The model under review builds one solid part; all positions refer to its coordinate system, in mm. A direction names the side the tool comes from. Round coordinates to 2 decimals unless told otherwise and drop trailing zeros. Order: outer loops, then holes, each group sorted by start corner. A loop starts at its lowest first (then second) coordinate and runs counter-clockwise, first axis right, second up. Notation, with made-up numbers: M 22.25,0 L 36.25,0 A17 cw 36.25,18 Z; hole C 81,37.5 d9. An arc over 180 degrees is marked long. Answer as a JSON object with one key per item and string values. Group by question number.
1) The part is to be moulded in two halves that separate along X. For faces 1 (the flat face through (-26.358, -0.239, 43.368)), 2 (the flat face through (27.625, 0, 25)), 3 (the cylindrical face through (28.62, -23.45, 27.78)), 4 (the flat face through (28, 0, 0)), say which applies: +X half, -X half, draft (parallel to the pull), parting line (faces both ways), or undercut.
2) To check wall thickness, follow line 1 (X direction, y = 12, z = 36) (3 decimals); line 2 (X direction, y = -14, z = 46) (3 decimals); line 3 (Y direction, x = 25.5, z = 9). State the ranges of each line that lie inside material, in increasing order.
3) For faces 5 (the flat face through (14, 21, 52.3)), 6 (the flat face through (25.125, -22, 25)), 7 (the flat face through (26, 17.05, 25)), 8 (the flat face through (0, 0, 54.8)), list the 3-axis set-ups (+Z, -Z, +X, -X, +Y, -Y) from which the entire face can be reached by the end or side of a thin tool; tool diameter is ignored.
4) Consider section C-C, the plane x = -3. Write out the cut boundary in (y, z) (3 decimals).
5) Consider section B-B, the plane y = -11. Write out the cut boundary in (x, z) (3 decimals).
6) Insertion check: pin 1 Ø2 at (x, y) = (14, -21) entering from -Z; pin 2 Ø0.8 at (x, z) = (-26, 30.5) entering from +Y; pin 3 Ø2 at (x, y) = (13.5, 21.5) entering from -Z. Each pin has a flat end and moves straight along its axis. Give the tip position at first contact, or say it passes through.
Autodesk Inventor part; units mm, degrees
ref_plane "Work Plane1" through (-24.875, -24.875, 49.8) normal (0, 0, 1) x (1, 0, 0)
ref_plane "Work Plane2" through (-24.875, -24.875, 0) normal (0, 0, -1) x (0, 1, 0)
ref_plane "YZ Plane" through (0, 0, 0) normal (1, 0, 0) x (0, 1, 0)
sketch "Sketch1" plane through (0, 0, 0) normal (0, 0, 1) x (1, 0, 0)
  circle A0 centre (-21.9, -21.9) radius 1.875
  circle A1 centre (21.9, 21.9) radius 1.875
  circle A2 centre (21.9, -21.9) radius 1.875
  circle A3 centre (-21.9, 21.9) radius 1.875
  circle A4 centre (14.4, 20.8) radius 2.0734
  circle A5 centre (-14.4, -20.8) radius 2.0734
  circle A6 centre (14.4, -20.8) radius 2.0734
  circle A7 centre (20.8, -14.4) radius 2.0734
  line L0 (-17.05, 17.05) -> (-17.05, -17.05)
  line L1 (17.05, 17.05) -> (-17.05, 17.05)
  line L2 (17.05, -17.05) -> (17.05, 17.05)
  line L3 (-17.05, -17.05) -> (17.05, -17.05)
  circle A8 centre (20.8, 14.4) radius 2.0734
  circle A9 centre (-14.4, 20.8) radius 2.0734
  circle A10 centre (-20.8, -14.4) radius 2.0734
  circle A11 centre (-20.8, 14.4) radius 2.0734
  line L4 (-22.9, 24.875) -> (22.9, 24.875)
  arc A12 (-22.9, 24.875) -> (-24.875, 22.9) centre (-22.9, 22.9) ccw
  line L5 (-24.875, -22.9) -> (-24.875, 22.9)
  arc A13 (-24.875, -22.9) -> (-22.9, -24.875) centre (-22.9, -22.9) ccw
  line L6 (22.9, -24.875) -> (-22.9, -24.875)
  arc A14 (22.9, -24.875) -> (24.875, -22.9) centre (22.9, -22.9) ccw
  line L7 (24.875, 22.9) -> (24.875, -22.9)
  arc A15 (24.875, 22.9) -> (22.9, 24.875) centre (22.9, 22.9) ccw
  line L8 (-24.875, 24.875) -> (24.875, 24.875)
  line L9 (24.875, 24.875) -> (24.875, -24.875)
  line L10 (24.875, -24.875) -> (-24.875, -24.875)
  line L11 (-24.875, -24.875) -> (-24.875, 24.875)
  line L12 (-24.875, 24.875) -> (24.875, -24.875) construction
  line L13 (24.875, 24.875) -> (-24.875, -24.875) construction
  point P0 (0, 0)
ref_plane "Work Plane1" through (-24.875, -24.875, 49.8) normal (0, 0, 1) x (1, 0, 0)
extrude "Extrusion1" add sketch "Sketch1" along normal blind 5 from surface at 49.8 contours A0 | A1 | A2 | A3 | A4 | A5 | A6 | A7 | L1 L2 L3 L0 | A8 | A9 | A10 | A11 | L4 A15 L7 A14 L6 A13 L5 A12 | A12 L11 L8 | L8 L9 A15 | A13 L10 L11 | L9 L10 A14
sketch "Sketch2" plane through (-24.875, 24.875, 54.8) normal (0, 0, 1) x (1, 0, 0)
  line L0 (49.75, 0) -> (49.75, -49.75)
  line L1 (0, 0) -> (49.75, 0)
  line L2 (0, -49.75) -> (0, 0)
  line L3 (49.75, -49.75) -> (0, -49.75)
  line L4 (49.75, -49.75) -> (50, -49.75)
  line L5 (50, -49.75) -> (50, 0)
  line L6 (50, 0) -> (49.75, 0)
  line L7 (49.75, 0) -> (49.75, -49.75)
  line L8 (50, -49.75) -> (55, -49.75)
  line L9 (55, -49.75) -> (55, 0)
  line L10 (55, 0) -> (50, 0)
  line L11 (50, 0) -> (50, -49.75)
  line L12 (24.875, -49.75) -> (24.875, 0)
  line L13 (0, 0) -> (0, -49.75)
  line L14 (0, -49.75) -> (-0.25, -49.75)
  line L15 (-0.25, -49.75) -> (-0.25, 0)
  line L16 (-0.25, 0) -> (0, 0)
  line L17 (0, 0) -> (0, -49.75)
  line L18 (-0.25, -49.75) -> (-5.25, -49.75)
  line L19 (-5.25, -49.75) -> (-5.25, 0)
  line L20 (-5.25, 0) -> (-0.25, 0)
  line L21 (-0.25, 0) -> (-0.25, -49.75)
  point P0 (24.875, -24.875)
  point P1 (-0.25, 0)
  point P2 (50, 0)
  point P3 (50, 0)
  point P4 (-0.25, 0)
  dimension "d2" = 0.25
  dimension "d3" = 49.75
  dimension "d4" = 5
  dimension "d5" = 49.75
extrude "Extrusion2" add sketch "Sketch2" against normal blind 5 contours L6 L5 L4 L0 | L10 L9 L8 L5 | L2 L14 L15 L16 | L15 L18 L19 L20
ref_plane "Work Plane2" through (-24.875, -24.875, 0) normal (0, 0, -1) x (0, 1, 0)
extrude "Extrusion3" add sketch "Sketch2" against normal up to surface (54.8 mm away) contours L10 L9 L8 L5 | L15 L18 L19 L20
sketch "Sketch3" plane through (25.125, -24.875, 49.8) normal (-1, 0, 0) x (0, 0, 1)
  line L0 (-7.7, 7.825) -> (-42.1, 7.825)
  line L1 (-42.1, 41.925) -> (-7.7, 41.925)
  line L2 (-24.9, 7.825) -> (-24.9, 41.925)
  line L3 (-42.1, 7.825) -> (-7.7, 7.825)
  line L4 (-7.7, 7.825) -> (-7.7, 41.925)
  line L5 (-7.7, 41.925) -> (-42.1, 41.925)
  line L6 (-42.1, 41.925) -> (-42.1, 7.825)
  line L7 (-42.1, 7.825) -> (-7.7, 41.925) construction
  line L8 (-7.7, 7.825) -> (-42.1, 41.925) construction
  point P0 (-49.8, 24.875)
  point P1 (-24.9, 24.875)
extrude "Extrusion4" cut sketch "Sketch3" against normal blind 2.5
mirror "Mirror1" about plane through (0, 0, 0) normal (1, 0, 0) of "Extrusion4"
sketch "Sketch4" plane through (25.125, -24.875, 49.8) normal (0, 0, -1) x (-1, 0, 0)
  circle A0 centre (47.025, 2.975) radius 1.875
  circle A1 centre (3.225, 46.775) radius 1.875
  circle A2 centre (3.225, 2.975) radius 1.875
  circle A3 centre (47.025, 46.775) radius 1.875
  circle A4 centre (10.725, 45.675) radius 2.0734
  circle A5 centre (39.525, 4.075) radius 2.0734
  circle A6 centre (10.725, 4.075) radius 2.0734
  circle A7 centre (4.325, 10.475) radius 2.0734
  line L0 (42.175, 41.925) -> (42.175, 7.825)
  line L1 (8.075, 41.925) -> (42.175, 41.925)
  line L2 (8.075, 7.825) -> (8.075, 41.925)
  line L3 (42.175, 7.825) -> (8.075, 7.825)
  circle A8 centre (4.325, 39.275) radius 2.0734
  circle A9 centre (39.525, 45.675) radius 2.0734
  circle A10 centre (45.925, 10.475) radius 2.0734
  circle A11 centre (45.925, 39.275) radius 2.0734
  line L4 (48.025, 49.75) -> (2.225, 49.75)
  arc A12 (50, 47.775) -> (48.025, 49.75) centre (48.025, 47.775) ccw
  line L5 (50, 1.975) -> (50, 47.775)
  arc A13 (48.025, 0) -> (50, 1.975) centre (48.025, 1.975) ccw
  line L6 (2.225, 0) -> (48.025, 0)
  arc A14 (0.25, 1.975) -> (2.225, 0) centre (2.225, 1.975) ccw
  line L7 (0.25, 47.775) -> (0.25, 1.975)
  arc A15 (2.225, 49.75) -> (0.25, 47.775) centre (2.225, 47.775) ccw
  point P0 (25.125, 24.875)
extrude "Extrusion5" cut sketch "Sketch4" against normal blind 2.5 contours A4 | A5 | A6 | L0 L3 L2 L1 | A9
chamfer "Chamfer1" distance 2.5 angle 45 8 edges at (-25.125, 0, 42.1) (-25.125, 0, 7.7) (25.125, 0, 42.1) (25.125, 0, 7.7) (0, 17.05, 49.8) (17.05, 0, 49.8) (-17.05, 0, 49.8) (0, -17.05, 49.8)
fillet "Fillet1" radius 5 4 edges at (30.125, -24.875, 27.4) (-30.125, -24.875, 27.4) (-30.125, 24.875, 27.4) (30.125, 24.875, 27.4)
properties part number "Cover Top (Full)"
Results list:
{
 "1": {"face 1": "undercut", "face 2": "undercut", "face 3": "+X half", "face 4": "draft"},
 "2": {"line 1": "-30.125 to -27.625, 27.625 to 30.125", "line 2": "-30.125 to -25.125, 25.125 to 30.125", "line 3": "-24.86 to -17.05, 17.05 to 24.86"},
 "3": {"face 5": "-Z", "face 6": "-Z, +Y, -Y", "face 7": "none", "face 8": "+Z, +X, -X, +Y, -Y"},
 "4": {"outline": "M -24.875,49.8 L -19.55,49.8 L -17.05,52.3 L 17.05,52.3 L 19.55,49.8 L 24.875,49.8 L 24.875,54.8 L -24.875,54.8 Z"},
 "5": {"outline": "M -30.125,0 L -25.125,0 L -25.125,5.2 L -27.625,7.7 L -27.625,42.1 L -25.125,44.6 L -25.125,49.8 L -19.55,49.8 L -17.05,52.3 L 17.05,52.3 L 19.55,49.8 L 25.125,49.8 L 25.125,44.6 L 27.625,42.1 L 27.625,7.7 L 25.125,5.2 L 25.125,0 L 30.125,0 L 30.125,54.8 L -30.125,54.8 Z"},
 "6": {"pin 1": "z = 52.3", "pin 2": "y = 24.85", "pin 3": "z = 49.8"}
}
